Here's the drawing with two shaded views (mm, measured from the low corner). I have some questions. Coordinates: 2 decimals unless noted, no trailing zeros. Loops run counter-clockwise (first coordinate to the right, second up) from the corner with the lowest first, then second, coordinate; pieces in that order, holes last. Notation, with made-up numbers: (-21.5, 40.25) - (-15.5, 40.25) arc R12 cw to (-15.5, 51.25) - close; hole circle Ø3 at (32.5, 19). An arc over 180 degrees is marked (long way). Use a Markdown table: item, result.
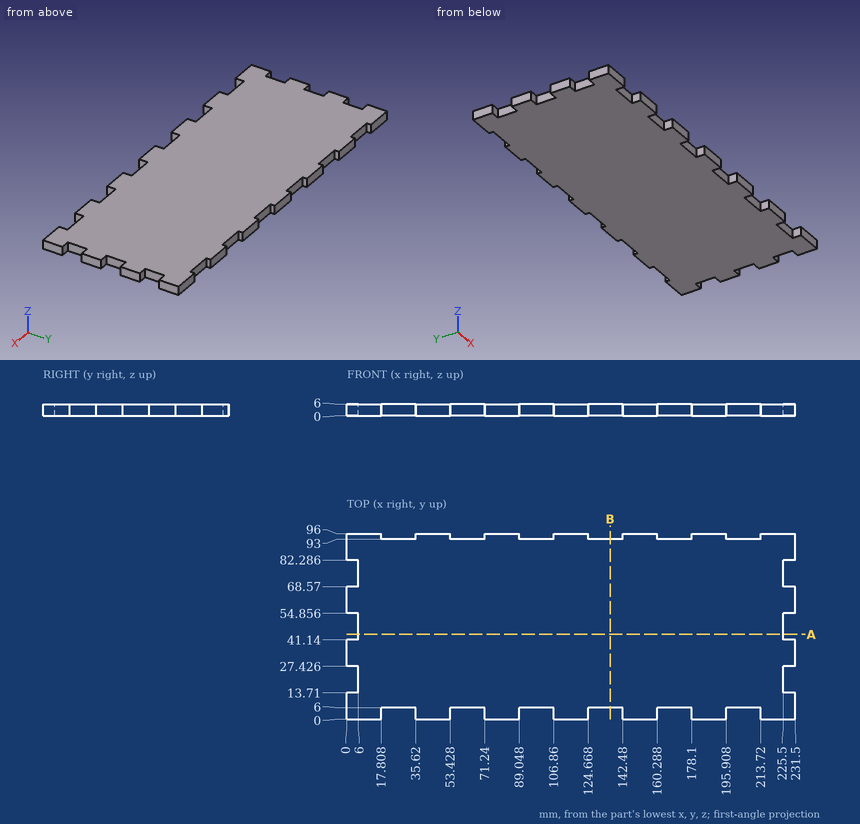
Q1. Will these pins go through, and if not, where does the flat tip stop? P1, Ø1, axis at y = 43, z = 3.5, coming from the +X side; P2, Ø1.8, axis at x = 94, z = 2.5, coming from the +Y side; P3, Ø1, axis at y = 74, z = 5, coming from the -X side.
Check values:
| item | result |
|---|---|
| P1 | x = 225.5 |
| P2 | y = 93 |
| P3 | x = 6 |
Q2. I want a section at B-B, the plane x = 136. Write out the boundary of the cut face in (y, z).
Check values:
| item | result |
|---|---|
| outline | (6, 0) - (93, 0) - (93, 6) - (6, 6) - close |
Q3. Please list where these lines run through material, in increasing order: L1, parallel to Y at x = 138, z = 0.95; L2, parallel to X at y = 24, z = 2.6. Write a range as from..to.
Check values:
| item | result |
|---|---|
| L1 | 6..93 |
| L2 | 6..225.5 |
Q4. I want a section at A-A, the plane y = 44. Write out the boundary of the cut face in (x, z), then the cut area to 3 significant figures.
Check values:
| item | result |
|---|---|
| outline | (6, 0) - (225.5, 0) - (225.5, 6) - (6, 6) - close |
| area | 1,320 mm^2 |
